```python
from build123d import *

# Parameters (mm, degrees)
F_5_8_0_625_DIAMETER_HOLE1_D     = 15.875
F_5_8_0_625_DIAMETER_HOLE1_DEPTH = 25.4
F_5_8_0_625_DIAMETER_HOLE1_TIP   = 4.769331164
CUT_EXTRUDE1_DEPTH               = 45.165608085
CUT_EXTRUDE1_DEPTH_BACK          = 45.165608085
SKETCH3_W                        = 31.75
SKETCH3_H                        = 0.79375
F_6_CLEARANCE_HOLE1_D            = 3.6576
CHAMFER1_SIZE                    = 1.5875


with BuildPart() as part:
    # Sketch1 → Revolve1 (revolve)
    with BuildSketch(Plane(origin=(0, 0, 0), x_dir=(1, 0, 0), z_dir=(0, 1, 0)), mode=Mode.PRIVATE) as revolve1_sk:
        Polygon((0, 0), (7.9375, 0), (11.1125, 0), (11.1125, 31.75), (3.175, 31.75), (3.175, 41.275), (0, 41.275), (0, 25.4), align=None)
    revolve(revolve1_sk.sketch.rotate(Axis((0, 0, -25.4), (0, 0, 1)), 180), axis=Axis((0, 0, -25.4), (0, 0, 1)))

    # 5/8 (0.625) Diameter Hole1
    with Locations(Plane.XY):
        with Locations((0, 0)):
            Hole(F_5_8_0_625_DIAMETER_HOLE1_D / 2, depth=F_5_8_0_625_DIAMETER_HOLE1_DEPTH)
            with Locations((0, 0, -(F_5_8_0_625_DIAMETER_HOLE1_DEPTH + F_5_8_0_625_DIAMETER_HOLE1_TIP / 2))):  # 118° drill point
                Cone(0, F_5_8_0_625_DIAMETER_HOLE1_D / 2, F_5_8_0_625_DIAMETER_HOLE1_TIP, mode=Mode.SUBTRACT)

    # Sketch3 → Cut-Extrude1 (cut, two sides: drawn at the far end of the back side and taken through both)
    with BuildSketch(Plane(origin=(0, 0, 0), x_dir=(0, 0, -1), z_dir=(1, 0, 0)).offset(-CUT_EXTRUDE1_DEPTH_BACK)):
        with Locations((15.875, 10.715625)):
            Rectangle(SKETCH3_W, SKETCH3_H)
    extrude(amount=CUT_EXTRUDE1_DEPTH + CUT_EXTRUDE1_DEPTH_BACK, mode=Mode.SUBTRACT)

    # #6 Clearance Hole1 (through all)
    with Locations(Plane(origin=(0, 10.31875, 0), x_dir=(1, 0, 0), z_dir=(0, 1, 0))):
        with Locations((0, 5.08)):
            Hole(F_6_CLEARANCE_HOLE1_D / 2)

    # Chamfer1
    chamfer1_edges = [part.edges().sort_by_distance(p)[0] for p in [
        (7.9375, 0, 0),
    ]]
    chamfer(chamfer1_edges, length=CHAMFER1_SIZE)


solid = part.part
```
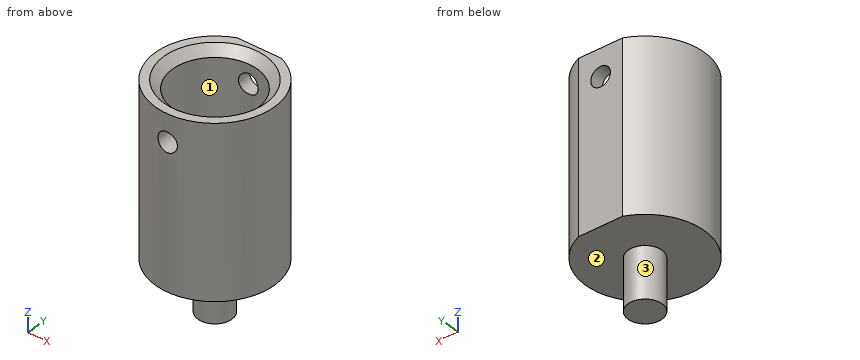
Geometry: final body of the model. Coordinates: model frame, mm. Face numbers are marked on the shaded views. Coordinates: 2 decimals unless noted, no trailing zeros. Order: outer loops, then holes, each group sorted by start corner. A loop starts at its lowest first (then second) coordinate and runs counter-clockwise, first axis right, second up. Notation, with made-up numbers: (-25, 40) -> (26, 40) arc R18 cw to (26, 73) -> close; hole circle Ø1 at (-24, 41). An arc over 180 degrees is marked (long way). Write each question's results on one line, items separated by ' | '. Start each with the question number.
1) Cut plane A-A, the plane z = -5.08. Output: boundary loops of the cut face in (x, y) (1 decimal).
2) Material intervals for line 1 along Y through (x, z) = (0, -17.75); line 2 along Z through (x, y) = (0, -9.8); line 3 along X through (y, z) = (0, -6.75), sorted ascending.
3) Mould query, pull axis Y, two halves, no side actions, for the marked faces 1, 2 and 3. Classes: released by +Y, released by -Y, zero draft, split by the parting line, or undercut.
4) Cut plane B-B, the plane z = -34. Output: boundary loops of the cut face in (x, y) (3 decimals), and give its area (3 significant figures).
5) First-contact query: pin 1 (1 mm diameter, centred on y = -7, z = -22, fed in from +X); pin 2 (8 mm diameter, centred on y = -6, z = -20, fed in from +X); pin 3 (3.5 mm diameter, centred on x = 0, z = -5.08, fed in from +Y); pin 4 (6 mm diameter, centred on x = -3, y = 5.5, fed in from -Z). Flat tips, straight axial feed; report the tip coordinate or a pass-through.
Checks:
1) outline: (-4.1, 10.3) arc R11.1 ccw to (-1.8, -11) -> (-1.8, -7.7) arc R7.9 cw to (-1.8, 7.7) -> (-1.8, 10.3) -> close; (1.8, -11) arc R11.1 ccw to (4.1, 10.3) -> (1.8, 10.3) -> (1.8, 7.7) arc R7.9 cw to (1.8, -7.7) -> close
2) line 1: -11.11 to -7.94, 7.94 to 10.32 | line 2: -31.75 to -6.91, -3.25 to 0 | line 3: -11.11 to -7.94, 7.94 to 11.11
3) face 1: undercut | face 2: zero draft | face 3: split by the parting line
4) outline: circle Ø6.35 at (0, 0) | area: 31.7 mm^2
5) pin 1: x = 9.01 | pin 2: x = 10.93 | pin 3: through | pin 4: z = -31.75
